Could you check a few things on this model? Use its own coordinates, in mm. A direction names the side the tool comes from. Round coordinates to 2 decimals unless told otherwise and drop trailing zeros. Order: outer loops, then holes, each group sorted by start corner. A loop starts at its lowest first (then second) coordinate and runs counter-clockwise, first axis right, second up.
Autodesk Inventor part; units mm, degrees
ref_plane "Work Plane1" through (20.3835, 0, 0) normal (-1, 0, 0) x (0, 1, 0)
ref_plane "Work Plane2" through (0, 20.3835, 0) normal (0, -1, 0) x (-1, 0, 0)
ref_plane "YZ Plane" through (0, 0, 0) normal (1, 0, 0) x (0, 1, 0)
sketch "Sketch1" plane through (0, 0, 0) normal (0, 0, 1) x (1, 0, 0)
  circle A0 centre (0, 0) radius 20.3835
  dimension "d0" = 40.767
extrude "Extrusion1" add sketch "Sketch1" against normal blind 101.6
sketch "Sketch11" plane through (0, 0, -101.6) normal (0, 0, -1) x (-1, 0, 0)
  circle A0 centre (0, 0) radius 20.3835
  line L0 (0, 20.3835) -> (-10.8843, 20.3835)
sketch "Sketch10" plane through (0, 0, 0) normal (0, 0, 1) x (1, 0, 0)
  circle A0 centre (0, 0) radius 20.3835
  line L0 (0, 20.3835) -> (-22.4405, 20.3835)
sketch "Sketch2" plane through (0, 0, 0) normal (0, 0, 1) x (1, 0, 0)
  circle A0 centre (0, 0) radius 20.3835
  line L0 (20.3835, 0) -> (20.3835, 20.3835)
sketch "Sketch3" plane through (0, 0, -101.6) normal (0, 0, -1) x (-1, 0, 0)
  circle A0 centre (0, 0) radius 20.3835
  line L0 (-20.3835, 0) -> (-20.3835, 20.3835)
ref_plane "Work Plane1" through (20.3835, 0, 0) normal (-1, 0, 0) x (0, 1, 0)
ref_plane "Work Plane2" through (0, 20.3835, 0) normal (0, -1, 0) x (-1, 0, 0)
sketch "Sketch4" plane through (20.3835, 0, 0) normal (-1, 0, 0) x (0, 1, 0)
  line L0 (20.3835, 101.6) -> (-20.3835, 101.6)
  circle A0 centre (0, 50.8) radius 20.3835
  line L1 (-20.3835, 0) -> (-20.3835, 101.6)
  point P0 (0, 0)
extrude "Extrusion2" add sketch "Sketch4" against normal blind 30.4165
extrude "Extrusion3" add sketch "Sketch4" along normal blind 20.3835
sketch "Sketch12" plane through (0, 20.3835, 0) normal (0, -1, 0) x (-1, 0, 0)
  line L0 (-20.3835, 30.4165) -> (0, 50.8)
  circle A0 centre (0, 50.8) radius 20.3835
  point P0 (0, 0)
extrude "Extrusion9" add sketch "Sketch12" against normal blind 30.4165
extrude "Extrusion10" add sketch "Sketch12" along normal blind 20.3835
sketch "Sketch5" plane through (0, 0, 0) normal (0, 0, 1) x (1, 0, 0)
  circle A0 centre (0, 0) radius 16.7767
  dimension "d7" = 33.5534
sketch "Sketch6" plane through (0, 0, 0) normal (0, 0, 1) x (1, 0, 0)
  circle A0 centre (0, 0) radius 12.7
  dimension "d8" = 25.4
sketch "Sketch7" plane through (50.8, 0, -50.8) normal (1, 0, 0) x (0, 0, -1)
  circle A0 centre (0, 0) radius 16.7767
  point P0 (-50.8, 0)
  dimension "d9" = 33.5534
sketch "Sketch8" plane through (50.8, 0, -50.8) normal (1, 0, 0) x (0, 0, -1)
  circle A0 centre (0, 0) radius 12.7
  point P0 (-50.8, 0)
  dimension "d10" = 25.4
sketch "Sketch9" plane through (0, 0, -101.6) normal (0, 0, -1) x (-1, 0, 0)
  circle A0 centre (0, 0) radius 16.7767
  dimension "d11" = 33.5534
extrude "Extrusion4" cut sketch "Sketch9" against normal blind 31.75
extrude "Extrusion5" cut sketch "Sketch7" against normal blind 31.75
extrude "Extrusion6" cut sketch "Sketch5" against normal blind 31.75
extrude "Extrusion7" cut sketch "Sketch6" against normal blind 101.6
extrude "Extrusion8" cut sketch "Sketch8" against normal blind 50.8
sketch "Sketch13" plane through (0, 50.8, -50.8) normal (0, 1, 0) x (1, 0, 0)
  circle A0 centre (0, 0) radius 16.7767
  point P0 (0, -50.8)
  dimension "d26" = 33.5534
extrude "Extrusion11" cut sketch "Sketch13" against normal blind 31.75
sketch "Sketch14" plane through (0, 50.8, -50.8) normal (0, 1, 0) x (1, 0, 0)
  line L0 (0, 0) -> (20.3835, -20.3835)
  circle A0 centre (0, 0) radius 12.7
  point P0 (0, -50.8)
  point P1 (14.4133, -14.4133)
  dimension "d29" = 25.4
extrude "Extrusion12" cut sketch "Sketch14" against normal blind 50.8
properties part number "4-way Tee 1 Inch"
Q1. We'd pull the mould along Z, two halves only. Please class faces 1 (the cylindrical face through (-16, 5.04, -85.95)), 2 (the flat face through (19.05, 13, -48)), 3 (the flat face through (-17, -3, -101.6)): released by +Z, released by -Z, zero draft, split by the parting line, or undercut.
Q2. For faces 4 (the flat face through (-13, 19.05, -55)), 5 (the flat face through (-3, 13, -31.75)), 6 (the cylindrical face through (13.89, -12.4, -48.05)), which set-ups out of +Z, -Z, +X, -X, +Y, -Y let a thin tool reach every point of the face, with its end or its side?
Q3. Imagine slicing it at C-C, the plane y = -9. Please give me the cut outline in (x, z), then the cut area to 3 significant figures.
Q4. Imagine slicing it at D-D, the plane z = -29. Please give me the cut outline in (x, y), then the cut area to 3 significant figures.
Q5. Imagine slicing it at A-A, the plane z = -50.8. Please give me the cut outline in (x, y), then the cut area to 3 significant figures.
Q6. Imagine slicing it at B-B, the plane x = 6. State how many separate pieces and enclosed holes the cut face has, then the cut area to 3 significant figures.
Q7. I need wall thicknesses on L1, parallel to Y at x = 30, z = -50; L2, parallel to Y at x = 13, z = -50; L3, parallel to Z at x = 0, y = 15.25. Which ranges of each line are inside material? Lowest first, please.
Q8. For P1, Ø23, axis at x = 0, z = -50.8, coming from the +Y side; P2, Ø15, axis at y = 0, z = -50.8, coming from the +X side; P3, Ø8, axis at y = 26.5, z = -22, coming from the +X side; P4, Ø17, axis at y = 0, z = -56, coming from the +X side, each with a flat end and sliding along its axis, tell me the tip position at first contact or that it passes through.
Filled in:
1. face 1: zero draft
1. face 2: undercut
1. face 3: released by -Z
2. face 4: +Y
2. face 5: +Z
2. face 6: +X
3. outline: (-18.29, -101.6) - (-14.16, -101.6) - (-14.16, -69.85) - (-8.96, -69.85) - (-8.96, -31.75) - (-14.16, -31.75) - (-14.16, 0) - (-18.29, 0) - close; (8.96, -69.85) - (14.16, -69.85) - (14.16, -101.6) - (18.29, -101.6) - (18.29, -69.09) - (50.8, -69.09) - (50.8, -64.96) - (19.05, -64.96) - (19.05, -59.76) - (8.96, -59.76) - close; (8.96, -41.84) - (19.05, -41.84) - (19.05, -36.64) - (50.8, -36.64) - (50.8, -32.51) - (18.29, -32.51) - (18.29, 0) - (14.16, 0) - (14.16, -31.75) - (8.96, -31.75) - close
3. area: 1,340 mm2
4. outline: circle Ø40.77 at (0, 0); hole circle Ø33.55 at (0, 0)
4. area: 421 mm2
5. outline: (-20.38, 0) arc R20.38 ccw to (0, -20.38) - (50.8, -20.38) - (50.8, -16.78) - (19.05, -16.78) - (19.05, -12.7) - (0, -12.7) arc R12.7 cw to (-12.7, 0) - (-12.7, 19.05) - (-16.78, 19.05) - (-16.78, 50.8) - (-20.38, 50.8) - close; (12.7, 12.7) - (19.05, 12.7) - (19.05, 16.78) - (50.8, 16.78) - (50.8, 20.38) - (20.38, 20.38) - (20.38, 50.8) - (16.78, 50.8) - (16.78, 19.05) - (12.7, 19.05) - close
5. area: 989 mm2
6. separate pieces: 3
6. enclosed holes: 0
6. area: 1,160 mm2
7. L1: y = -20.37 to -16.76, 16.76 to 20.37
7. L2: y = -20.37 to -12.67, 12.67 to 19.05
7. L3: z = -69.85 to -63.5, -38.1 to -31.75
8. P1: stops at y = -5.39
8. P2: stops at x = -10.25
8. P3: passes through
8. P4: stops at x = 19.05
